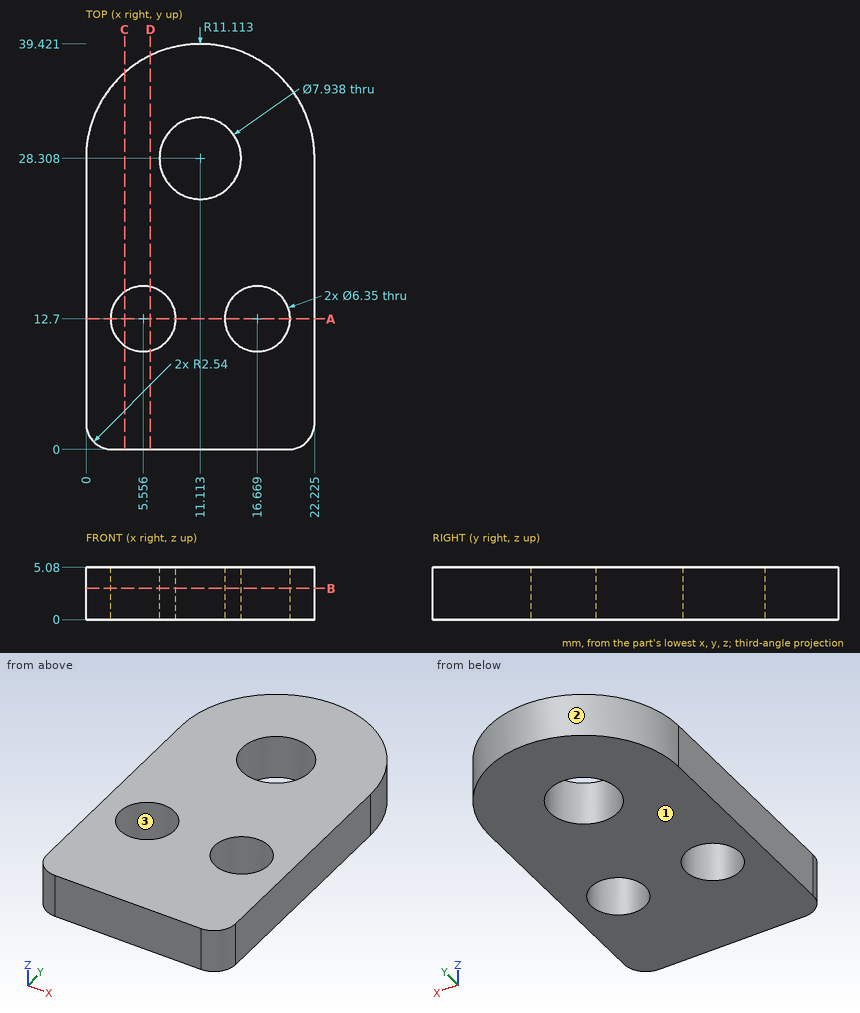
Answer from the drawing. Dimensions are ordinates in mm from the lowest x, y and z of the part. Round coordinates to 2 decimals unless told otherwise and drop trailing zeros. Loops run counter-clockwise (first coordinate to the right, second up) from the corner with the lowest first, then second, coordinate; pieces in that order, holes last.
Q1. Section A-A on y = 12.7 is taken. Write down the section's boundary in (x, z) (1 decimal).
Q2. Consider probe 1 along X at (y, z) = (11.5, 4.7) (1 decimal); probe 2 along X at (y, z) = (10, 3.85) (1 decimal); probe 3 along Y at (x, z) = (5.5, 1.3) (1 decimal). Determine where each line is inside the solid, lowest interval first.
Q3. Determine the mould class of the marked faces 1, 2 and 3 for opening direction X: released by +X, released by -X, zero draft, split by the parting line, or undercut.
Q4. Section C-C on x = 3.75 is taken. Write down the section's boundary in (y, z).
Q5. Section D-D on x = 6.25 is taken. Write down the section's boundary in (y, z).
Q6. Section B-B on z = 3.05 is taken. Give the number of separate pieces and of enclosed holes in the cut face.
Output:
1. outline: (0, 0) - (2.4, 0) - (2.4, 5.1) - (0, 5.1) - close; (8.7, 0) - (13.5, 0) - (13.5, 5.1) - (8.7, 5.1) - close; (19.8, 0) - (22.2, 0) - (22.2, 5.1) - (19.8, 5.1) - close
2. probe 1: x = 0 to 2.6, 8.5 to 13.7, 19.6 to 22.2
2. probe 2: x = 0 to 3.9, 7.2 to 15, 18.3 to 22.2
2. probe 3: y = 0 to 9.5, 15.9 to 37.9
3. face 1: zero draft
3. face 2: split by the parting line
3. face 3: undercut
4. outline: (0, 0) - (10.09, 0) - (10.09, 5.08) - (0, 5.08) - close; (15.31, 0) - (36.63, 0) - (36.63, 5.08) - (15.31, 5.08) - close
5. outline: (0, 0) - (9.6, 0) - (9.6, 5.08) - (0, 5.08) - close; (15.8, 0) - (38.3, 0) - (38.3, 5.08) - (15.8, 5.08) - close
6. separate pieces: 1
6. enclosed holes: 3
